Verification items for the finished model (mm, model axes). Face numbers are marked on the shaded views. A direction names the side the tool comes from. Coordinates: 2 decimals unless noted, no trailing zeros. Write each loop counter-clockwise with the first axis right and the second up, starting at its lowest first coordinate (ties: lowest second). Pieces come first, ordered by that corner, then holes. Notation, with made-up numbers: (57.5, -19) -> (62.5, -19) arc R18 ccw to (62.5, -1) -> close; hole circle Ø8 at (80.5, 47). An arc over 180 degrees is marked (long way). Answer in a Markdown table with one row per item.
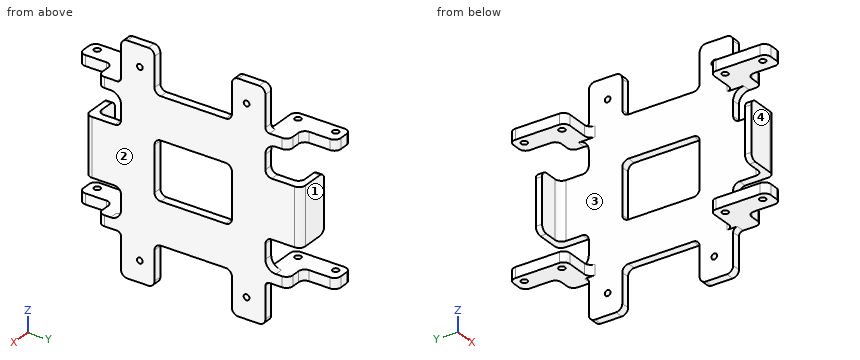
```python
from build123d import *

# Parameters (mm, degrees)
BOSS_EXTRUDE4_DEPTH = 4
BOSS_EXTRUDE5_DEPTH = 5
FILLET5_R           = 5
FILLET6_R           = 2
FILLET7_R           = 3
SKETCH11_R          = 1.5
CUT_EXTRUDE6_DEPTH  = 104.181370521
SKETCH12_R          = 1.368026344
SKETCH12_R_2        = 1.35
CUT_EXTRUDE7_DEPTH  = 5
FILLET8_R           = 3
SKETCH13_W          = 27.5
SKETCH13_H          = 3
BOSS_EXTRUDE6_DEPTH = 12
FILLET9_R           = 3
SKETCH14_W          = 20
SKETCH14_H          = 18.5
BOSS_EXTRUDE7_DEPTH = 4
FILLET10_R          = 3


with BuildPart() as part:
    # Sketch9 → Boss-Extrude4 (new body)
    with BuildSketch(Plane.ZY.offset(-47.264100781)):
        Polygon((-107.5, -0.5), (-67.5, -0.5), (-67.5, -17.5), (-40, -17.5), (-40, -0.5), (0, -0.5), (0, 15.5), (-107.5, 15.5), align=None)
    extrude(amount=BOSS_EXTRUDE4_DEPTH)

    # Sketch10 → Boss-Extrude5 (add)
    with BuildSketch(Plane(origin=(0, 0, -20), x_dir=(-1, 0, 0), z_dir=(0, 0, -1))):
        Polygon((-43.264100781, -0.5), (-27.264100781, -0.5), (-27.264100781, -27.5), (-37.264100781, -27.5), (-37.264100781, -11.5), (-47.264100781, -11.5), (-47.264100781, 7.5), (-43.264100781, 7.5), align=None)
    boss_extrude5 = extrude(amount=BOSS_EXTRUDE5_DEPTH)

    # Mirror1: Boss-Extrude5 across plane
    add(boss_extrude5.mirror(Plane.XY.offset(-53.75)))

    # Fillet5
    fillet5_edges = [part.edges().sort_by_distance(p)[0] for p in [
        (45.264100781, -0.5, -25),
        (45.264100781, -0.5, -82.5),
    ]]
    fillet(fillet5_edges, radius=FILLET5_R)

    # Fillet6
    fillet6_edges = [part.edges().sort_by_distance(p)[0] for p in [
        (45.264100781, -0.5, -20),
        (45.264100781, -0.5, -87.5),
    ]]
    fillet(fillet6_edges, radius=FILLET6_R)

    # Fillet7
    fillet7_edges = [part.edges().sort_by_distance(p)[0] for p in [
        (43.264100781, -0.5, -85),
        (37.264100781, -11.5, -85),
        (37.264100781, -11.5, -22.5),
        (43.264100781, -0.5, -22.5),
    ]]
    fillet(fillet7_edges, radius=FILLET7_R)
    fillet7_2_edges = [part.edges().sort_by_distance(p)[0] for p in [
        (45.264100781, 15.5, -107.5),
        (45.264100781, -0.5, -107.5),
        (45.264100781, 15.5, 0),
        (47.264100781, -11.5, -85),
        (27.264100781, -0.5, -85),
        (37.264100781, -27.5, -85),
        (27.264100781, -27.5, -85),
        (47.264100781, -11.5, -22.5),
        (27.264100781, -0.5, -22.5),
        (37.264100781, -27.5, -22.5),
        (27.264100781, -27.5, -22.5),
        (45.264100781, -0.5, 0),
    ]]
    fillet(fillet7_2_edges, radius=FILLET7_R)

    # Sketch11 → Cut-Extrude6 (cut, through all)
    with BuildSketch(Plane(origin=(0, 0, -87.5), x_dir=(-1, 0, 0), z_dir=(0, 0, -1))):
        with Locations((-31.264100781, -5)):
            Circle(SKETCH11_R)
        with Locations((-31.264100781, -23)):
            Circle(SKETCH11_R)
    extrude(amount=-CUT_EXTRUDE6_DEPTH, mode=Mode.SUBTRACT)

    # Sketch12 → Cut-Extrude7 (cut)
    with BuildSketch(Plane.ZY.offset(-43.264100781)):
        with Locations(Location((-97.5, 8.5, 0), (0, 0, 270))):
            Circle(SKETCH12_R)
        with Locations(Location((-10, 8.5, 0), (0, 0, 270))):
            Circle(SKETCH12_R_2)
    extrude(amount=-CUT_EXTRUDE7_DEPTH, mode=Mode.SUBTRACT)

    # Fillet8
    fillet8_edges = [part.edges().sort_by_distance(p)[0] for p in [
        (45.264100781, -0.5, -40),
        (45.264100781, -0.5, -67.5),
    ]]
    fillet(fillet8_edges, radius=FILLET8_R)

    # Sketch13 → Boss-Extrude6 (add)
    with BuildSketch(Plane.ZY.offset(-43.264100781)):
        with Locations((-53.75, -16)):
            Rectangle(SKETCH13_W, SKETCH13_H)
    extrude(amount=BOSS_EXTRUDE6_DEPTH)

    # Fillet9
    fillet9_edges = [part.edges().sort_by_distance(p)[0] for p in [
        (43.264100781, -14.5, -53.75),
        (31.264100781, -16, -40),
        (31.264100781, -16, -67.5),
        (47.264100781, -17.5, -53.75),
    ]]
    fillet(fillet9_edges, radius=FILLET9_R)

    # Sketch14 → Boss-Extrude7 (add)
    with BuildSketch(Plane.ZY.offset(-47.264100781)):
        with Locations((-30, 24.75)):
            Rectangle(SKETCH14_W, SKETCH14_H)
        with Locations((-77.5, 24.75)):
            Rectangle(SKETCH14_W, SKETCH14_H)
    extrude(amount=BOSS_EXTRUDE7_DEPTH)

    # Fillet10
    fillet10_edges = [part.edges().sort_by_distance(p)[0] for p in [
        (45.264100781, 15.5, -20),
        (45.264100781, 15.5, -40),
        (45.264100781, 15.5, -67.5),
        (45.264100781, 15.5, -87.5),
    ]]
    fillet(fillet10_edges, radius=FILLET10_R)

    # Mirror2: part across plane


with BuildPart() as part_1:
    add(part.part)
    add(part.part.mirror(Plane(origin=(43.264100781, 34, -20), x_dir=(0, 0, 1), z_dir=(0, -1, 0))))


solid = part_1.part
```
1. Sectioned sample at D-D, the plane y = 91. Record the cut outline in (x, z), and give its area (3 significant figures).
Findings below:
| item | result |
|---|---|
| outline | (27.26, -87.5) -> (29.76, -87.5) -> (29.76, -82.5) -> (27.26, -82.5) -> close; (27.26, -25) -> (29.76, -25) -> (29.76, -20) -> (27.26, -20) -> close; (32.76, -87.5) -> (37.26, -87.5) -> (37.26, -82.5) -> (32.76, -82.5) -> close; (32.76, -25) -> (37.26, -25) -> (37.26, -20) -> (32.76, -20) -> close |
| area | 70.0 mm² |
2. Sectioned sample at A-A, the plane y = 35. Record the cut outline in (x, z).
Findings below:
| item | result |
|---|---|
| outline | (43.26, -87.5) -> (47.26, -87.5) -> (47.26, -67.5) -> (43.26, -67.5) -> close; (43.26, -40) -> (47.26, -40) -> (47.26, -20) -> (43.26, -20) -> close |
3. Access from +Z, -Z, +X, -X, +Y, -Y to the whole of each face (thin tool, end or side, straight path). Record for the marked faces 1, 2, 3 and 4.
Findings below:
| item | result |
|---|---|
| face 1 | +X, -X, +Y |
| face 2 | +Z, -Z, +X, +Y, -Y |
| face 3 | -X |
| face 4 | +X, -X, -Y |
4. Sectioned sample at C-C, the plane y = 8.5. Record the cut outline in (x, z), and give its area (3 significant figures).
Findings below:
| item | result |
|---|---|
| outline | (43.26, -107.5) -> (47.26, -107.5) -> (47.26, -98.87) -> (43.26, -98.87) -> close; (43.26, -96.13) -> (47.26, -96.13) -> (47.26, -11.35) -> (43.26, -11.35) -> close; (43.26, -8.65) -> (47.26, -8.65) -> (47.26, 0) -> (43.26, 0) -> close |
| area | 408 mm² |
5. Material ranges on probe 1 along Z at (x, y) = (44.7, 8.5); probe 2 along Z at (x, y) = (32.5, -12.5); probe 3 along X at (y, z) = (73, -22.35), recorded low to high. Write a range as from..to.
Findings below:
| item | result |
|---|---|
| probe 1 | z = -107.5..-98.87, -96.13..-11.35, -8.65..0 |
| probe 2 | z = -87.5..-82.5, -25..-20 |
| probe 3 | x = 27.26..29.76, 32.76..47.26 |
6. Sectioned sample at B-B, the plane z = -97.5. Record the cut outline in (x, y), and give its area (3 significant figures).
Findings below:
| item | result |
|---|---|
| outline | (43.26, -0.5) -> (47.26, -0.5) -> (47.26, 7.13) -> (43.26, 7.13) -> close; (43.26, 9.87) -> (47.26, 9.87) -> (47.26, 15.5) -> (43.26, 15.5) -> close; (43.26, 52.5) -> (47.26, 52.5) -> (47.26, 58.13) -> (43.26, 58.13) -> close; (43.26, 60.87) -> (47.26, 60.87) -> (47.26, 68.5) -> (43.26, 68.5) -> close |
| area | 106 mm² |
7. Go/stop test with flat-tipped pins: pin 1 (2 mm diameter, centred on x = 46, y = 29, fed in from -Z); pin 2 (3.5 mm diameter, centred on y = 84, z = -55.5, fed in from -X); pin 3 (2 mm diameter, centred on x = 43, z = -14, fed in from -Y). Record where each tip stops, or that it passes through.
Findings below:
| item | result |
|---|---|
| pin 1 | stops at z = -87.5 |
| pin 2 | stops at x = 31.26 |
| pin 3 | stops at y = -0.5 |
